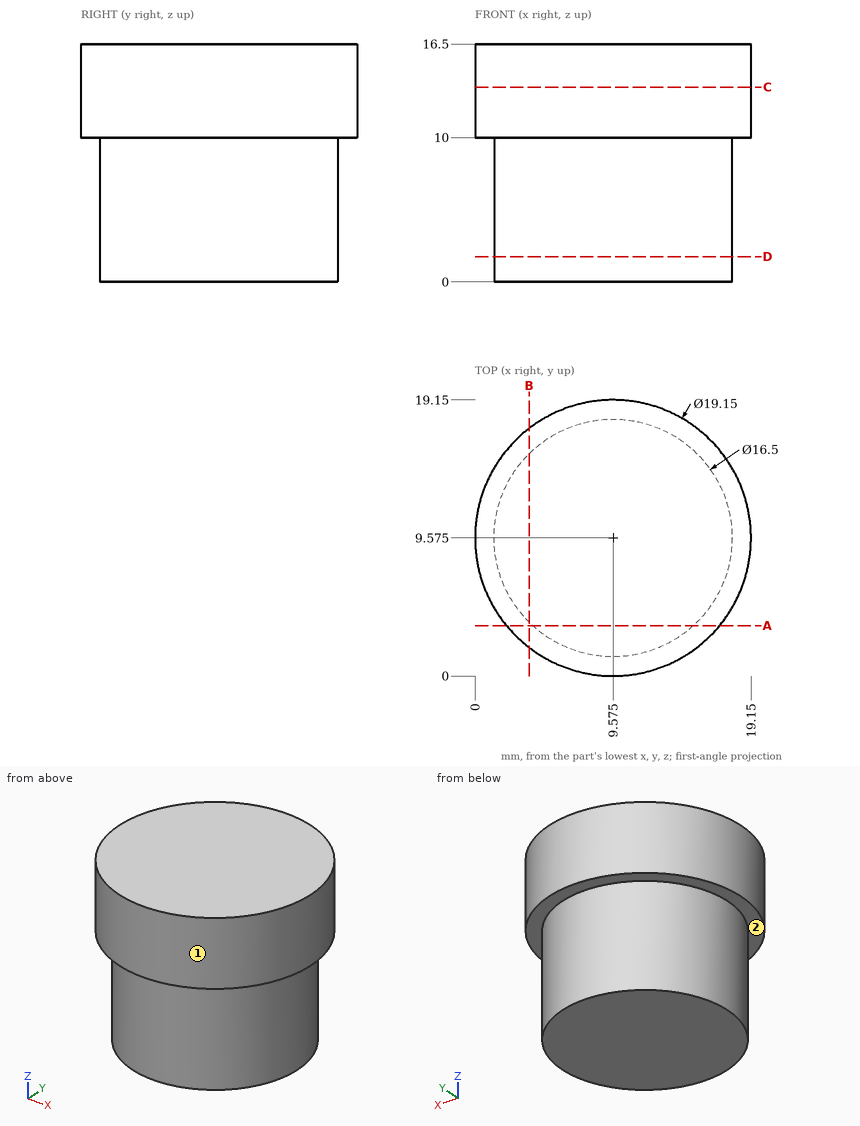
Can you work these out from the drawing? Everything is in mm from the part's minimum corner. A direction names the side the tool comes from. Coordinates: 2 decimals unless noted, no trailing zeros. Loops run counter-clockwise (first coordinate to the right, second up) from the corner with the lowest first, then second, coordinate; pieces in that order, holes last.
1) Will these pins go through, and if not, where does the flat tip stop? pin 1 Ø4 at (x, z) = (9, 7.5) entering from -Y (3 decimals); pin 2 Ø2 at (y, z) = (17, 12.5) entering from -X.
Reported:
pin 1: stops at y = 1.325
pin 2: stops at x = 2.48
2) Which directions (+Z, -Z, +X, -X, +Y, -Y) give clear straight access to the entire face, cutting with the end or side of a thin tool? Please do the marked faces 1 and 2.
Reported:
face 1: +Z, -Z
face 2: -Z
3) Imagine slicing it at A-A (y = 3.5). List the corners of the cut face in (x, z) for me.
Reported:
outline: (2.17, 10) - (3.99, 10) - (3.99, 0) - (15.16, 0) - (15.16, 10) - (16.98, 10) - (16.98, 16.5) - (2.17, 16.5) - close
4) Please list where these lines run through material, in increasing order: line 1 along X through (y, z) = (9.5, 9.75); line 2 along Z through (x, y) = (16.75, 15.5); line 3 along Y through (x, z) = (10.75, 9.5).
Reported:
line 1: x = 1.33 to 17.82
line 2: z = 10 to 16.5
line 3: y = 1.41 to 17.74
5) Imagine slicing it at B-B (x = 3.75). List the corners of the cut face in (y, z) for me.
Reported:
outline: (1.98, 10) - (3.73, 10) - (3.73, 0) - (15.42, 0) - (15.42, 10) - (17.17, 10) - (17.17, 16.5) - (1.98, 16.5) - close
6) Imagine slicing it at C-C (z = 13.5). List the corners of the cut face in (x, y) for me (3 decimals).
Reported:
outline: circle Ø19.15 at (9.575, 9.575)
7) Imagine slicing it at D-D (z = 1.75). List the corners of the cut face in (x, y) for me (3 decimals), and give its area (3 significant figures).
Reported:
outline: circle Ø16.5 at (9.575, 9.575)
area: 214 mm2
